The listing builds one solid part. Answer for the finished solid, in the listing's coordinates (mm). A direction names the side the tool comes from. Give positions to 0.01 mm unless a question says otherwise; leave off trailing zeros. Write each loop counter-clockwise with the first axis right and the second up, starting at its lowest first coordinate (ties: lowest second). Pieces come first, ordered by that corner, then holes. Notation, with made-up numbers: (-27.75, 16.5) - (13.25, 16.5) arc R14 cw to (13.25, 21.5) - close; hole circle Ø5 at (-20, 36.5). An arc over 180 degrees is marked (long way). One line per item, written item: value. Start each with the question number.
from build123d import *

# Parameters (mm, degrees)
F0_W      = 50.8
F0_H      = 304.8
F1_DEPTH  = 50.8
F2_W      = 63.5
F2_H      = 50.8
F3_DEPTH  = 6.35
F4_R      = 7.94131
F4_R_2    = 7.9375
F5_DEPTH  = 6.35
F6_R      = 7.9375
F7_DEPTH  = 50.8
F8_W      = 63.5
F8_H      = 50.8
F9_DEPTH  = 6.35
F10_R     = 7.9375
F11_DEPTH = 6.35


with BuildPart() as f1:
    # F0 (on Top) → F1 (new body)
    with BuildSketch(Plane.XY):
        with Locations((-25.4, -152.4)):
            Rectangle(F0_W, F0_H)
    extrude(amount=F1_DEPTH)

    # F2 (on face) → F3 (join)
    with BuildSketch(Plane(origin=(-50.8, 0, 0), x_dir=(0, -1, 0), z_dir=(-1, 0, 0))):
        Polygon((-88.9, 0), (0, 0), (0, 50.8), (63.5, 50.8), (63.5, 152.4), (-88.9, 152.4), align=None)
        with Locations((31.75, 25.4)):
            Rectangle(F2_W, F2_H)
    extrude(amount=F3_DEPTH)

    # F4 (on face) → F5 (cut)
    with BuildSketch(Plane(origin=(-57.15, 0, 0), x_dir=(0, -1, 0), z_dir=(-1, 0, 0))):
        with Locations((-50.8, 127)):
            Circle(F4_R)
        with Locations((-50.8, 25.4)):
            Circle(F4_R_2)
    extrude(amount=-F5_DEPTH, mode=Mode.SUBTRACT)

    # F6 (on face) → F7 (cut)
    with BuildSketch(Plane(origin=(-50.8, 0, 0), x_dir=(0, -1, 0), z_dir=(-1, 0, 0))):
        with Locations((228.6, 25.4)):
            Circle(F6_R)
    extrude(amount=-F7_DEPTH, mode=Mode.SUBTRACT)

    # F8 (on face) → F9 (join)
    with BuildSketch(Plane.YZ):
        with Locations((-31.75, 25.4)):
            Rectangle(F8_W, F8_H)
        Polygon((0, 50.8), (0, 0), (88.9, 0), (88.9, 152.4), (-63.5, 152.4), (-63.5, 50.8), align=None)
    extrude(amount=F9_DEPTH)

    # F10 (on face) → F11 (cut)
    with BuildSketch(Plane.YZ.offset(6.35)):
        with Locations((50.8, 127)):
            Circle(F10_R)
        with Locations((50.8, 25.4)):
            Circle(F10_R)
    extrude(amount=-F11_DEPTH, mode=Mode.SUBTRACT)


solid = f1.part
Item 1: For faces 1 (the flat face through (0, -186, 25)), 2 (the flat face through (-26, 0, 25)), 3 (the flat face through (-26, -150, 50.8)), 4 (the flat face through (-50.8, 14, 94)), determine the directions among +Z, -Z, +X, -X, +Y, -Y from which every point of the face is accessible in a straight line to the end or side of a thin tool.
Item 2: Find section B-B on y = 50.8. Determine the outline of the cut face in (x, z), plus the area to 3 significant figures.
Item 3: Find section D-D on x = -4. Determine the outline of the cut face in (y, z) (1 decimal).
Item 4: Find section A-A on z = 127. Determine the outline of the cut face in (x, y).
Item 5: Straight lines are drawn through the part: line 1 along Z through (x, y) = (5.25, 50.8); line 2 along X through (y, z) = (59, 142); line 3 along X through (y, z) = (-142, 46). For each, find the intervals that lie inside material, in ascending order.
Item 6: The mould has two halves that part along Y. Classify faces 5 (the cylindrical face through (3.22, 42.87, 25.75)), 6 (the flat face through (6.35, 12, 77)), 7 (the flat face through (-26, -304.8, 25)): +Y half, -Y half, draft (parallel to the pull), parting line (faces both ways), or undercut.
Item 7: Each of these flat-tipped pins is pushed along its axis until it touches: pin 1 Ø15 at (y, z) = (-171, 13.5) entering from +X; pin 2 Ø15 at (x, y) = (-32.5, -151.5) entering from +Z; pin 3 Ø20.5 at (y, z) = (50.8, 127) entering from -X; pin 4 Ø15 at (x, z) = (-15.5, 13) entering from +Y. Where does it stop, or does it pass through?
Item 8: Find section C-C on z = 64. Determine the outline of the cut face in (x, y).
Values:
1. face 1: +Z, -Z, +X, -Y
1. face 2: +Z, -Z, +Y
1. face 3: +Z, +Y, -Y
1. face 4: +Z, +Y
2. outline: (-57.15, 0) - (-50.8, 0) - (-50.8, 17.46) - (-57.15, 17.46) - close; (-57.15, 33.34) - (-50.8, 33.34) - (-50.8, 119.06) - (-57.15, 119.06) - close; (-57.15, 134.94) - (-50.8, 134.94) - (-50.8, 152.4) - (-57.15, 152.4) - close; (0, 0) - (6.35, 0) - (6.35, 17.46) - (0, 17.46) - close; (0, 33.34) - (6.35, 33.34) - (6.35, 119.06) - (0, 119.06) - close; (0, 134.94) - (6.35, 134.94) - (6.35, 152.4) - (0, 152.4) - close
2. area: 1,530 mm^2
3. outline: (-304.8, 0) - (0, 0) - (0, 50.8) - (-304.8, 50.8) - close; hole circle Ø15.9 at (-228.6, 25.4)
4. outline: (-57.15, -63.5) - (-50.8, -63.5) - (-50.8, 42.86) - (-57.15, 42.86) - close; (-57.15, 58.74) - (-50.8, 58.74) - (-50.8, 88.9) - (-57.15, 88.9) - close; (0, -63.5) - (6.35, -63.5) - (6.35, 42.86) - (0, 42.86) - close; (0, 58.74) - (6.35, 58.74) - (6.35, 88.9) - (0, 88.9) - close
5. line 1: 0 to 17.46, 33.34 to 119.06, 134.94 to 152.4
5. line 2: -57.15 to -50.8, 0 to 6.35
5. line 3: -50.8 to 0
6. face 5: undercut
6. face 6: draft
6. face 7: -Y half
7. pin 1: x = 0
7. pin 2: z = 50.8
7. pin 3: x = -57.15
7. pin 4: y = 0
8. outline: (-57.15, -63.5) - (-50.8, -63.5) - (-50.8, 88.9) - (-57.15, 88.9) - close; (0, -63.5) - (6.35, -63.5) - (6.35, 88.9) - (0, 88.9) - close
